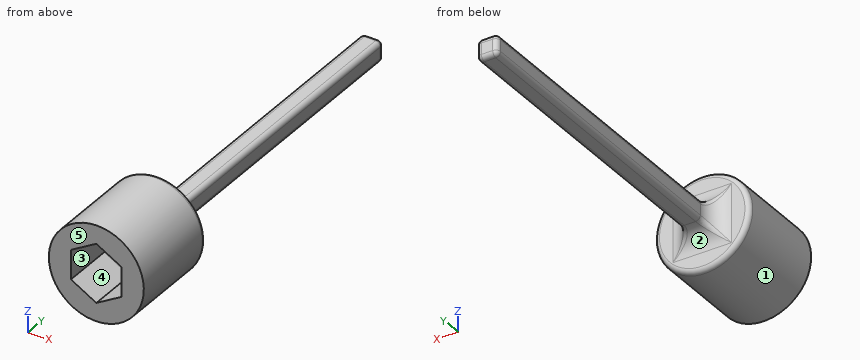
```python
from build123d import *

# Parameters (mm, degrees)
SKETCH1_R           = 6.35
BOSS_EXTRUDE1_DEPTH = 12.7
SKETCH2_W           = 2.778125
SKETCH2_H           = 2.778125
BOSS_EXTRUDE2_DEPTH = 44.45
FILLET1_R           = 2.54
FILLET2_R           = 0.635
CUT_EXTRUDE1_DEPTH  = 10.033
FILLET3_R           = 3.175


with BuildPart() as part:
    # Sketch1 → Boss-Extrude1 (new body)
    with BuildSketch(Plane(origin=(0, 0, 0), x_dir=(0, 0, -1), z_dir=(0, 1, 0))):
        with Locations(Location((0, 0, 0), (0, 0, 180))):
            Circle(SKETCH1_R)
    extrude(amount=BOSS_EXTRUDE1_DEPTH)

    # Sketch2 → Boss-Extrude2 (add)
    with BuildSketch(Plane(origin=(-12.7, 12.7, 0), x_dir=(0, 0, -1), z_dir=(0, -1, 0))):
        with Locations((0, 12.7)):
            Rectangle(SKETCH2_W, SKETCH2_H)
    extrude(amount=-BOSS_EXTRUDE2_DEPTH)

    # Fillet1
    fillet1_edges = [part.edges().sort_by_distance(p)[0] for p in [
        (0, 12.7, -1.3890625),
        (-1.3890625, 12.7, 0),
        (1.3890625, 12.7, 0),
        (0, 12.7, 1.3890625),
    ]]
    fillet(fillet1_edges, radius=FILLET1_R)

    # Fillet2
    fillet2_edges = [part.edges().sort_by_distance(p)[0] for p in [
        (2.288098275, 13.301228117, -2.288098275),
        (-2.288098218, 13.301228166, -2.288098218),
        (2.288098215, 13.301228168, 2.288098215),
        (-2.288098198, 13.301228182, 2.288098198),
        (0, 12.7, -6.35),
        (1.3890625, 36.195, -1.3890625),
        (-1.3890625, 36.195, -1.3890625),
        (0, 57.15, 1.3890625),
        (-1.3890625, 36.195, 1.3890625),
        (1.3890625, 57.15, 0),
        (1.3890625, 36.195, 1.3890625),
        (0, 57.15, -1.3890625),
        (-1.3890625, 57.15, 0),
    ]]
    fillet(fillet2_edges, radius=FILLET2_R)

    # Sketch3 → Cut-Extrude1 (cut)
    with BuildSketch(Plane.XZ):
        Polygon((-3.3909, 1.957737028), (-3.3909, -1.957737028), (0, -3.915474056), (3.3909, -1.957737028), (3.3909, 1.957737028), (0, 3.915474056), align=None)
    extrude(amount=-CUT_EXTRUDE1_DEPTH, mode=Mode.SUBTRACT)

    # Fillet3
    fillet3_edges = [part.edges().sort_by_distance(p)[0] for p in [
        (-1.69545, 10.033, 2.936605542),
        (1.69545, 10.033, 2.936605542),
        (3.3909, 10.033, 0),
        (1.69545, 10.033, -2.936605542),
        (-1.69545, 10.033, -2.936605542),
        (-3.3909, 10.033, 0),
    ]]
    fillet(fillet3_edges, radius=FILLET3_R)


solid = part.part
```
Read the model definition and answer for the solid it produces. Units are mm, in the model's axes. Face numbers are marked on the shaded views. A direction names the side the tool comes from. Give positions to 0.01 mm unless a question says otherwise; leave off trailing zeros. Write each loop counter-clockwise with the first axis right and the second up, starting at its lowest first coordinate (ties: lowest second). Pieces come first, ordered by that corner, then holes. Notation, with made-up numbers: M -36.75,-28.75 L 16.25,-28.75 A24 ccw 16.25,-2.75 Z; hole C 16,47.5 d11. An arc over 180 degrees is marked long. Put each result on its own line as item: value. Start each with the question number.
1. Which of the six approach directions +Z, -Z, +X, -X, +Y, -Y give full straight-line access (tool end or side, diameter ignored) to the marked faces 4 and 5?
2. Consider line 1 along X through (y, z) = (36, 0.75); line 2 along Y through (x, z) = (-4.25, 2.25); line 3 along Y through (x, z) = (3.5, 5). Determine where each line is inside the solid, lowest interval first.
3. Each of these flat-tipped pins is pushed along its axis until it touches: pin 1 Ø6 at (x, y) = (3.5, 26) entering from +Z; pin 2 Ø3 at (x, y) = (1, 18) entering from -Z; pin 3 Ø1.2 at (y, z) = (42.5, 0) entering from +X. Where does it stop, or does it pass through?
4. The part is cut by section A-A, the plane y = 5.5. Give the vertices of the cut face in (x, z).
5. The part is cut by section B-B, the plane y = 50.5. Give the vertices of the cut face in (x, z) (3 decimals), and give its area (3 significant figures).
6. For a pull along Z with two mould halves and no side action, classify the marked faces 1, 2 and 3 as released by +Z, released by -Z, zero draft, split by the parting line, or undercut.
Final values:
1. face 4: -Y
1. face 5: +Z, -Z, +X, -X, -Y
2. line 1: x = -1.39 to 1.39
2. line 2: y = 0 to 12.7
2. line 3: y = 0 to 12.57
3. pin 1: stops at z = 1.39
3. pin 2: stops at z = -1.39
3. pin 3: stops at x = 1.39
4. outline: C 0,0 d12.7; hole M -3.39,-1.96 L 0,-3.92 L 3.39,-1.96 L 3.39,1.96 L 0,3.92 L -3.39,1.96 Z
5. outline: M -1.389,-0.754 A0.635 ccw -0.754,-1.389 L 0.754,-1.389 A0.635 ccw 1.389,-0.754 L 1.389,0.754 A0.635 ccw 0.754,1.389 L -0.754,1.389 A0.635 ccw -1.389,0.754 Z
5. area: 7.37 mm²
6. face 1: split by the parting line
6. face 2: released by -Z
6. face 3: undercut
